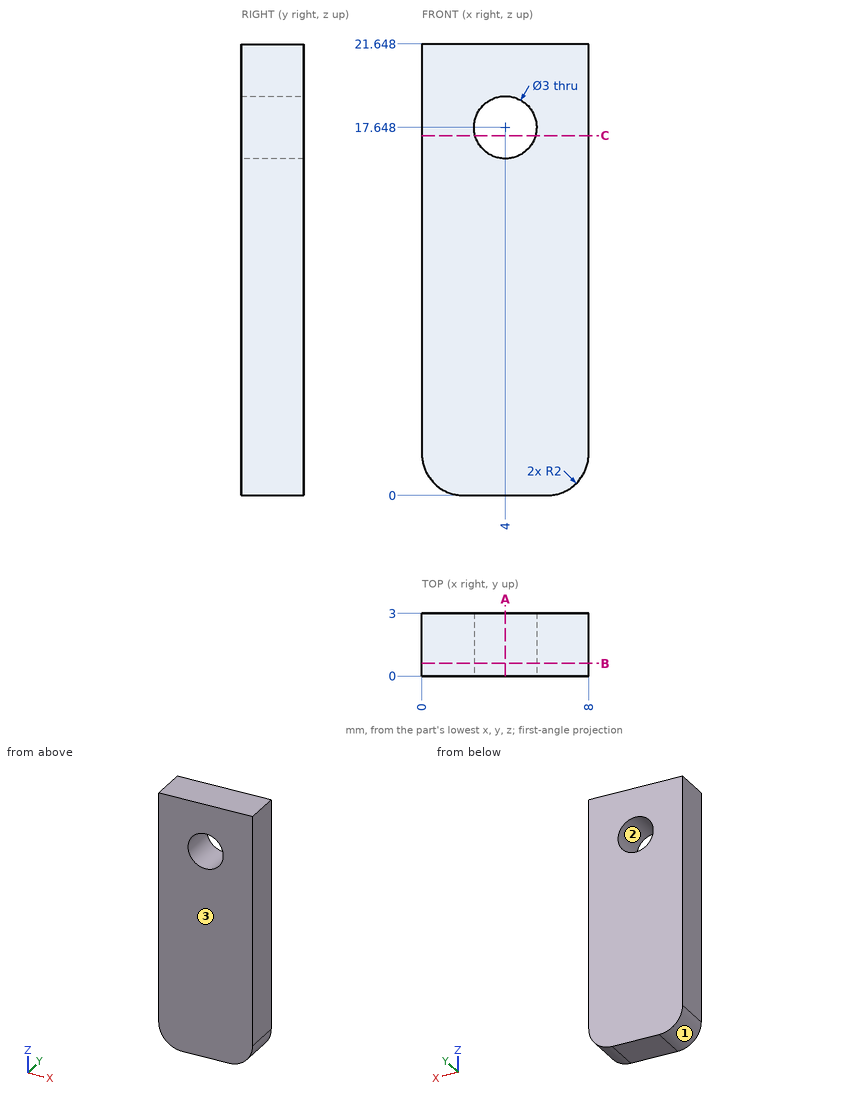
For this review, use the dimensioned drawing (mm, ordinates from the lowest corner) and the shaded views. Round coordinates to 2 decimals unless told otherwise and drop trailing zeros. Write each loop counter-clockwise with the first axis right and the second up, starting at its lowest first coordinate (ties: lowest second). Pieces come first, ordered by that corner, then holes. Notation, with made-up numbers: (15.5, 76.5) -> (68.5, 76.5) arc R35 ccw to (68.5, 112.5) -> close; hole circle Ø5 at (-21.75, 15). An arc over 180 degrees is marked (long way). Use one line per item in the form item = value.
Q1. To check wall thickness, follow probe 1 along X at (y, z) = (1.2, 18.25); probe 2 along X at (y, z) = (0.35, 18); probe 3 along Z at (x, y) = (1.5, 1.6). State the ranges of each line that lie inside material, in increasing order. Write a range as from..to.
Resolved:
probe_1 = 0..2.63, 5.37..8
probe_2 = 0..2.54, 5.46..8
probe_3 = 0.06..21.65
Q2. Consider section C-C (z = 17.25). State the section outline as (x, y) points.
Resolved:
outline = (0, 0) -> (2.55, 0) -> (2.55, 3) -> (0, 3) -> close; (5.45, 0) -> (8, 0) -> (8, 3) -> (5.45, 3) -> close
Q3. Consider section B-B (y = 0.6). State the section outline as (x, z) points.
Resolved:
outline = (0, 2) arc R2 ccw to (2, 0) -> (6, 0) arc R2 ccw to (8, 2) -> (8, 21.65) -> (0, 21.65) -> close; hole circle Ø3 at (4, 17.65)
Q4. Consider section A-A (x = 4). State the section outline as (y, z) points.
Resolved:
outline = (0, 0) -> (3, 0) -> (3, 16.15) -> (0, 16.15) -> close; (0, 19.15) -> (3, 19.15) -> (3, 21.65) -> (0, 21.65) -> close
Q5. Clearance check with a flat-ended pin moving along its axis: pin 1 Ø3.5 at (x, z) = (4, 17.65) entering from -Y. State where the tip first meets the part, or that it passes through.
Resolved:
pin_1 = 0
Q6. The part is to be moulded in two halves that separate along Z. For the marked faces 1, 2 and 3, say which applies: released by +Z, released by -Z, zero draft, split by the parting line, or undercut.
Resolved:
face_1 = released by -Z
face_2 = undercut
face_3 = zero draft
